from build123d import *

# Parameters (mm, degrees)
SKETCH1_R           = 16
SKETCH1_R_2         = 2.06
BOSS_EXTRUDE1_DEPTH = 2.5
CUT_EXTRUDE1_DEPTH  = 23.765104876


with BuildPart() as part:
    # Sketch1 → Boss-Extrude1 (new body)
    with BuildSketch(Plane(origin=(0, 0, 0), x_dir=(1, 0, 0), z_dir=(0, 1, 0))):
        with Locations(Location((0, 0, 0), (0, 0, 270))):
            Circle(SKETCH1_R)
        with Locations(Location((0, 0, 0), (0, 0, 270))):
            Circle(SKETCH1_R_2, mode=Mode.SUBTRACT)
        with BuildLine():
            Line((-3, 0), (-15, 0))
            ThreePointArc((-15, 0), (-4.8703472, -14.187308348), (11.837295753, -9.212948999))
            Line((11.837295753, -9.212948999), (0.858729732, -2.874470951))
            ThreePointArc((0.858729732, -2.874470951), (-1.792178954, -2.405845921), (-3, 0))
        make_face(mode=Mode.SUBTRACT)
        with BuildLine():
            Line((-11.837295753, 9.212948999), (-0.858729732, 2.874470951))
            ThreePointArc((-0.858729732, 2.874470951), (1.792178954, 2.405845921), (3, 0))
            Line((3, 0), (15, 0))
            ThreePointArc((15, 0), (4.8703472, 14.187308348), (-11.837295753, 9.212948999))
        make_face(mode=Mode.SUBTRACT)
    extrude(amount=BOSS_EXTRUDE1_DEPTH)

    # Sketch2 → Cut-Extrude1 (cut, through all)
    with BuildSketch(Plane(origin=(0, 2.5, 0), x_dir=(1, 0, 0), z_dir=(0, 1, 0))):
        with BuildLine():
            Line((1.108433193, 2.787718755), (0.761124126, 1.914233545))
            ThreePointArc((0.761124126, 1.914233545), (1.004470219, 1.798510378), (1.230629548, 1.652014199))
            Line((1.230629548, 1.652014199), (1.792178954, 2.405845921))
            ThreePointArc((1.792178954, 2.405845921), (1.462820707, 2.619189871), (1.108433193, 2.787718755))
        make_face()
    extrude(amount=-CUT_EXTRUDE1_DEPTH, mode=Mode.SUBTRACT)


solid = part.part
Could you check a few things on this model? Use its own coordinates, in mm. A direction names the side the tool comes from. Round coordinates to 2 decimals unless told otherwise and drop trailing zeros. Loops run counter-clockwise (first coordinate to the right, second up) from the corner with the lowest first, then second, coordinate; pieces in that order, holes last. Notation, with made-up numbers: (44.5, 2.25) - (78.5, 2.25) arc R12 ccw to (78.5, 13.25) - close; hole circle Ø2 at (5, 24.25). An arc over 180 degrees is marked (long way). Write item = value, one per line.
1) Imagine slicing it at A-A (x = 0). Please give me the cut outline in (y, z), and give its area (3 significant figures).
Computed:
outline = (0, -16) - (2.5, -16) - (2.5, -15) - (0, -15) - close; (0, -3) - (2.5, -3) - (2.5, -2.06) - (0, -2.06) - close; (0, 2.06) - (2.5, 2.06) - (2.5, 3) - (0, 3) - close; (0, 15) - (2.5, 15) - (2.5, 16) - (0, 16) - close
area = 9.70 mm2
2) I'm going to push flat-ended pins straight in: P1, Ø1.2, axis at x = -8, y = 1.5, coming from the +Z side; P2, Ø0.8, axis at x = 8.5, y = 1.5, coming from the -Z side; P3, Ø1.5, axis at x = -12.5, y = 2, coming from the -Z side. Where does each tip first touch, or does it pass through?
Computed:
P1 = 14.19
P2 = -13.8
P3 = -10.86
3) If we mould it in two halves opening along Z, with no side actions, what happens to faces 3 (the flat face through (-2, 2.5, -1)), 4 (the cylindrical face through (-15.62, 1.23, -3.47)), 5 (the flat face through (-9, 1, 0))? For each: pulls with the +Z half, pulls with the -Z half, needs draft (parallel to the pull), parting line crosses it, or undercut.
Computed:
face_3 = needs draft
face_4 = parting line crosses it
face_5 = undercut
4) On a 3-axis mill with a long thin cutter (end or side, diameter ignored), from which of +Z, -Z, +X, -X, +Y, -Y can I reach the whole of each face in a straight line? I mean faces 1 (the cylindrical face through (0, 1, -3)), 2 (the flat face through (-2, 0, -1)). Say none if no direction works.
Computed:
face_1 = +Y, -Y
face_2 = +Z, -Z, +X, -X, -Y
5) Imagine slicing it at C-C (y = 1.55). Please give me the cut outline in (x, z).
Computed:
outline = circle Ø32 at (0, 0); hole (-15, 0) - (-3, 0) arc R3 cw to (0.86, 2.87) - (11.84, 9.21) arc R15 ccw to start; hole (-11.84, -9.21) arc R15 ccw to (15, 0) - (3, 0) arc R3 cw to (1.79, -2.41) - (1.23, -1.65) arc R2.06 ccw (long way) to (0.76, -1.91) - (1.11, -2.79) arc R3 cw to (-0.86, -2.87) - close
6) Imagine slicing it at D-D (x = -4). Please give me the cut outline in (y, z), and give its area (3 significant figures).
Computed:
outline = (0, -15.49) - (2.5, -15.49) - (2.5, -14.46) - (0, -14.46) - close; (0, -4.69) - (2.5, -4.69) - (2.5, 0) - (0, 0) - close; (0, 14.46) - (2.5, 14.46) - (2.5, 15.49) - (0, 15.49) - close
area = 16.9 mm2
7) Imagine slicing it at B-B (z = -5.5). Please give me the cut outline in (x, y).
Computed:
outline = (-15.02, 0) - (-5.41, 0) - (-5.41, 2.5) - (-15.02, 2.5) - close; (13.96, 0) - (15.02, 0) - (15.02, 2.5) - (13.96, 2.5) - close
8) I need wall thicknesses on line 1 along Z through (x, y) = (-8, 1.85); line 2 along Z through (x, y) = (-4, 0.3); line 3 along X through (y, z) = (2, -12.5). Which ranges of each line are inside material? Lowest first, please. Write a range as from..to.
Computed:
line_1 = -13.86..-12.69, -7..0, 12.69..13.86
line_2 = -15.49..-14.46, -4.69..0, 14.46..15.49
line_3 = -9.99..-8.29, 8.29..9.99
